The listing builds one solid part. Answer for the finished solid, in the listing's coordinates (mm). Face numbers are marked on the shaded views. A direction names the side the tool comes from. Coordinates: 2 decimals unless noted, no trailing zeros. Order: outer loops, then holes, each group sorted by start corner. A loop starts at its lowest first (then second) coordinate and runs counter-clockwise, first axis right, second up. Notation, with made-up numbers: M 56,73.5 L 110,73.5 A18 ccw 110,81.5 Z; hole C 69.5,4 d4. An arc over 180 degrees is marked long. One line per item, written item: value. Start each with the question number.
Q1. Straight lines are drawn through the part: line 1 along X through (y, z) = (43.5, 22); line 2 along Y through (x, z) = (-3.5, 10.5); line 3 along Y through (x, z) = (27, 25). For each, find the intervals that lie inside material, in ascending order. Write a range as [from, to].
Q2. The part is cut by section C-C on x = -7. Give the vertices of the cut face in (y, z), then the cut area to 3 significant figures.
Q3. The part is cut by section B-B on z = 6. Give the vertices of the cut face in (x, y).
Q4. The part is cut by section A-A on x = 20. Give the vertices of the cut face in (y, z), then the cut area to 3 significant figures.
Q5. Determine the mould class of the marked faces 1, 2, 3 and 4 for opening direction Y: pulls with the +Y half, pulls with the -Y half, needs draft (parallel to the pull), parting line crosses it, or undercut.
Q6. Each of these flat-tipped pins is pushed along its axis until it touches: pin 1 Ø12 at (x, y) = (21, -28) entering from +Z; pin 2 Ø1.5 at (x, y) = (8.5, -28) entering from +Z; pin 3 Ø1.1 at (y, z) = (-44.5, 15.5) entering from +X; pin 4 Ø8 at (x, z) = (5.5, 31) entering from -Y. Where does it stop, or does it pass through?
Q7. For the marked faces 5 and 6, determine the directions among +Z, -Z, +X, -X, +Y, -Y from which every point of the face is accessible in a straight line to the end or side of a thin tool.
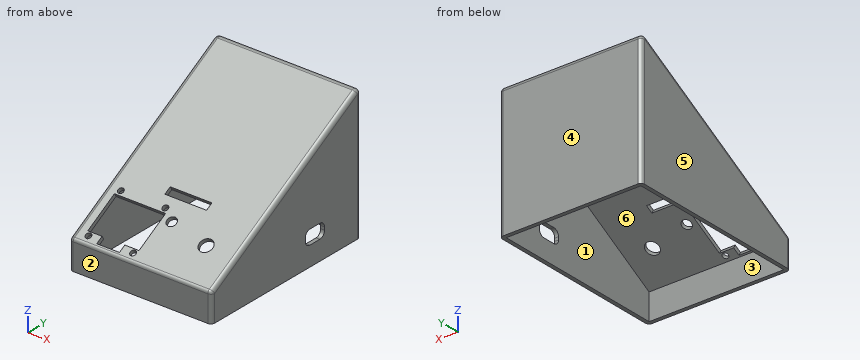
Autodesk Fusion 360 part; units mm, degrees
sketch "Sketch1" plane through (0, 0, 0) normal (0, 0, 1) x (1, 0, 0)
  line L0 (37.5, 48.5) -> (-37.5, 48.5)
  line L1 (-37.5, 48.5) -> (-37.5, -48.5)
  line L2 (-37.5, -48.5) -> (37.5, -48.5)
  line L3 (37.5, -48.5) -> (37.5, 48.5)
  line L4 (37.5, 48.5) -> (-37.5, -48.5) construction
  line L5 (-37.5, 48.5) -> (37.5, -48.5) construction
  dimension "d1" = 75
  dimension "d2" = 97
extrude "Extrude1" add sketch "Sketch1" along normal blind 15
sketch "Sketch2" plane through (37.5, 0, 0) normal (1, 0, 0) x (0, 1, 0)
  line L0 (-48.5, 0) -> (48.5, 0)
  line L1 (48.5, 0) -> (48.5, 15)
  line L2 (48.5, 15) -> (-48.5, 15)
  line L3 (-48.5, 15) -> (-48.5, 0)
  line L4 (-48.5, 15) -> (48.5, 71.003)
  line L5 (-48.5, 15) -> (74.9401, 15) construction
  line L6 (48.5, 71.003) -> (48.5, 15)
  dimension "d5" = 30
extrude "Extrude2" add sketch "Sketch2" against normal up to surface (75 mm away) contours L2 L4 L6
sketch "Sketch3" plane through (0, -18.6202, 32.2511) normal (0, -0.5, 0.866) x (1, 0, 0)
  line L0 (-37.5, 77.5037) -> (-37.5, -34.5022)
  line L1 (-37.5, -34.5022) -> (37.5, -34.5022)
  line L2 (37.5, -34.5022) -> (37.5, 77.5037)
  line L3 (37.5, 77.5037) -> (-37.5, 77.5037)
  line L4 (11, 3.5037) -> (-11, 3.5037)
  line L5 (-11, 3.5037) -> (-11, -0.4963)
  line L6 (-11, -0.4963) -> (11, -0.4963)
  line L7 (11, -0.4963) -> (11, 3.5037)
  line L8 (11, 3.5037) -> (-11, -0.4963) construction
  line L9 (-11, 3.5037) -> (11, -0.4963) construction
  line L10 (-32, -32.5022) -> (-5, -32.5022)
  line L11 (-5, -32.5022) -> (-5, -8.5022)
  line L12 (-5, -8.5022) -> (-32, -8.5022)
  line L13 (-32, -8.5022) -> (-32, -32.5022)
  circle A0 centre (-30.25, -6.2022) radius 1.5
  circle A1 centre (-6.75, -6.2022) radius 1.5
  circle A2 centre (21.25, -15.4993) radius 3.5
  line L14 (-32, -32.5022) -> (-24.5, -32.5022)
  line L15 (-24.5, -32.5022) -> (-24.5, -28.5022)
  line L16 (-24.5, -28.5022) -> (-32, -28.5022)
  line L17 (-32, -28.5022) -> (-32, -32.5022)
  line L18 (-5, -32.5022) -> (-12.5, -32.5022)
  line L19 (-12.5, -32.5022) -> (-12.5, -28.5022)
  line L20 (-12.5, -28.5022) -> (-5, -28.5022)
  line L21 (-5, -28.5022) -> (-5, -32.5022)
  circle A3 centre (-6.75, -30.5022) radius 1.5
  circle A4 centre (-30.25, -30.5022) radius 1.5
  line L22 (11, 3.5037) -> (37.5, 3.5037) construction
  line L23 (-11, 3.5037) -> (-37.5, 3.5037) construction
  line L24 (21.25, 3.5037) -> (21.25, -34.5022) construction
  circle A5 centre (0, -11.0022) radius 2.5
  line L25 (-5, -8.5022) -> (6, -8.5022) construction
  point P0 (0, 1.5037)
  dimension "d8" = 22
  dimension "d9" = 4
  dimension "d10" = 74
  dimension "d11" = 27
  dimension "d12" = 24
  dimension "d14" = 2
  dimension "d17" = 3
  dimension "d18" = 2.3
  dimension "d20" = 2.3
  dimension "d22" = 7
  dimension "d37" = 3
  dimension "d38" = 7.5
  dimension "d39" = 4
  dimension "d40" = 7.5
  dimension "d41" = 4
  dimension "d42" = 3
  dimension "d43" = 2
  dimension "d44" = 1.75
  dimension "d45" = 23.5
  dimension "d46" = 24.3
  dimension "d54" = 1.75
  dimension "d55" = 1.75
  dimension "d56" = 16.25
  dimension "d57" = 5
  dimension "d58" = 5
shell "Shell1" thickness 2 removed faces 1 at (-12.5, -16.1667, 0)
extrude "Extrude3" cut sketch "Sketch3" against normal blind 14 contours L4 L5 L6 L7 | L10 L11 L12 L13 L15 L16 L19 L20 | A0 | A1 | A2 | A3 | A4 | A5
sketch "Sketch4" plane through (37.5, 0, 0) normal (1, 0, 0) x (0, 1, 0)
  line L0 (-48.5, 0) -> (48.5, 0)
  line L1 (48.5, 0) -> (48.5, 71.003)
  line L2 (48.5, 71.003) -> (-48.5, 15)
  line L3 (-48.5, 15) -> (-48.5, 0)
sketch "Sketch5" plane through (37.5, 0, 0) normal (1, 0, 0) x (0, 1, 0)
  line L0 (15.5, 10.25) -> (22, 10.25)
  line L1 (25, 13.25) -> (25, 14.75)
  line L2 (22, 17.75) -> (15.5, 17.75)
  line L3 (12.5, 14.75) -> (12.5, 13.25)
  arc A0 (15.5, 17.75) -> (12.5, 14.75) centre (15.5, 14.75) ccw
  arc A1 (12.5, 13.25) -> (15.5, 10.25) centre (15.5, 13.25) ccw
  arc A2 (25, 14.75) -> (22, 17.75) centre (22, 14.75) ccw
  arc A3 (22, 10.25) -> (25, 13.25) centre (22, 13.25) ccw
  line L4 (18.75, 17.75) -> (18.75, 10.25) construction
  line L5 (12.5, 14) -> (25, 14) construction
  line L6 (-48.5, 0) -> (48.5, 0) construction
  line L7 (48.5, 0) -> (48.5, 71.003) construction
  point P0 (12.5, 10.25)
  point P1 (25, 10.25)
  point P2 (12.5, 17.75)
  dimension "d28" = 12.5
  dimension "d29" = 7.5
  dimension "d30" = 3
  dimension "d31" = 14
  dimension "d32" = 29.75
extrude "Extrude4" cut sketch "Sketch5" against normal blind 4
fillet "Fillet1" radius 2 8 edges at (0, 48.5, 71.003) (-37.5, 0, 43.0015) (0, -48.5, 15) (-37.5, -48.5, 7.5) (-37.5, 48.5, 35.5015) (37.5, 0, 43.0015) (37.5, -48.5, 7.5) (37.5, 48.5, 35.5015)
Output:
1. line 1: x = [-37.5, -35.5], [35.5, 37.5]
1. line 2: y = [-48.5, -46.5], [46.5, 48.5]
1. line 3: y = [-31.18, -27.18], [46.5, 48.5]
2. outline: M -48.5,0 L -46.5,0 L -46.5,13.85 L -45.32,14.53 L -46.32,16.26 L -47.5,15.58 A2 ccw -48.5,13.85 Z; M -43.76,17.74 L -42.76,16.01 L -42.3,16.27 L -43.3,18 Z; M -25.98,28 L -24.98,26.27 L -24.27,26.68 L -25.27,28.41 Z; M -22.71,29.89 L -21.71,28.16 L -18.05,30.27 L -19.05,32 Z; M -15.59,34 L -14.59,32.27 L 46.5,67.54 L 46.5,0 L 48.5,0 L 48.5,67.54 A2 ccw 45.5,69.27 Z
2. area: 324 mm^2
3. outline: M -37.5,-46.5 A2 ccw -35.5,-48.5 L 35.5,-48.5 A2 ccw 37.5,-46.5 L 37.5,46.5 A2 ccw 35.5,48.5 L -35.5,48.5 A2 ccw -37.5,46.5 Z; hole M -35.5,-46.5 L 35.5,-46.5 L 35.5,46.5 L -35.5,46.5 Z
4. outline: M -48.5,0 L -46.5,0 L -46.5,13.85 L -33.87,21.13 L -34.87,22.87 L -47.5,15.58 A2 ccw -48.5,13.85 Z; M -29.21,26.14 L -28.21,24.4 L 46.5,67.54 L 46.5,0 L 48.5,0 L 48.5,67.54 A2 ccw 45.5,69.27 Z
4. area: 371 mm^2
5. face 1: undercut
5. face 2: pulls with the -Y half
5. face 3: undercut
5. face 4: pulls with the +Y half
6. pin 1: stops at z = 30.3
6. pin 2: stops at z = 27.27
6. pin 3: stops at x = 37.5
6. pin 4: stops at y = -27.72
7. face 5: +Z, -Z, -X, +Y, -Y
7. face 6: -Z
